Geometry check sheet. Reference: the model listing, model coordinates, mm. A direction names the side the tool comes from. Round coordinates to 2 decimals unless told otherwise and drop trailing zeros. Write each loop counter-clockwise with the first axis right and the second up, starting at its lowest first coordinate (ties: lowest second). Pieces come first, ordered by that corner, then holes. Notation, with made-up numbers: M 34.5,51.5 L 88.5,51.5 A22 ccw 88.5,79.5 Z; hole C -2,2 d4. An arc over 180 degrees is marked long. Use a Markdown table: item, result.
Autodesk Inventor part; units mm, degrees
ref_plane "YZ Plane" through (0, 0, 0) normal (1, 0, 0) x (0, 1, 0)
ref_plane "XZ Plane" through (0, 0, 0) normal (0, 1, 0) x (-1, 0, 0)
ref_plane "XY Plane" through (0, 0, 0) normal (0, 0, 1) x (1, 0, 0)
ref_plane "Arbeitsebene9" through (-58.9003, 150.915, -19.5294) normal (1, 0, 0) x (0, 1, 0.0002861)
ref_plane "Arbeitsebene10" through (-3.3213, 95.2, -15) normal (1, 0, 0) x (0, 1, 0)
sketch "Skizze8" plane through (-3.3213, 95.2, -15) normal (1, 0, 0) x (0, 1, 0)
  line L0 (51.0327, -12.5388) -> (54.3913, -9.7235)
  line L1 (55.2125, -10.1069) -> (55.2018, -30.9624)
  line L2 (54.3802, -31.345) -> (51.0244, -28.5262)
  line L3 (50.2028, -28.9088) -> (50.1999, -34.5321)
  line L4 (50.2154, -4.5321) -> (50.2115, -12.1553)
  line L5 (50.2154, -13.2238) -> (55.2125, -9.0351)
  line L6 (55.2125, -9.0351) -> (55.2125, -32.0442)
  line L7 (55.2125, -32.0442) -> (50.2154, -27.8467)
  line L8 (50.2154, -13.2238) -> (50.2154, -27.8467)
  line L9 (54.9125, -9.678) -> (50.5154, -13.3638)
  line L10 (50.5154, -13.3638) -> (50.5154, -27.7069)
  line L11 (50.5154, -27.7069) -> (54.9125, -31.4004)
  line L12 (54.9125, -31.4004) -> (54.9125, -9.678)
  line L13 (50.5154, -13.3638) -> (46.5154, -13.3638)
  line L14 (50.5154, -13.3638) -> (54.5154, -13.3638) construction
  line L15 (46.5154, -13.3638) -> (46.5154, -27.7069)
  line L16 (46.5154, -27.7069) -> (50.5154, -27.7069)
  line L17 (67.5498, -4.541) -> (50.2154, -4.5321)
  line L18 (61.046, -34.5285) -> (50.2065, -34.5303)
  line L19 (46.5154, -13.3638) -> (49.8154, -13.3638)
  line L20 (49.8154, -13.3638) -> (49.8154, -4.5318)
  line L21 (49.8154, -4.5318) -> (46.5154, -4.5318)
  line L22 (46.5154, -4.5318) -> (46.5154, -13.3638)
  line L23 (46.5154, -27.7069) -> (49.8154, -27.7069)
  line L24 (49.8154, -27.7069) -> (49.8154, -34.5304)
  line L25 (49.8154, -34.5304) -> (46.5154, -34.5304)
  line L26 (46.5154, -34.5304) -> (46.5154, -27.7069)
  point P0 (-95.2, 15)
  point P1 (50.2154, -27.7069)
  point P2 (54.3913, -9.7235)
  point P3 (50.2154, -13.3638)
  dimension "d62" = 0.3
  dimension "d63" = 4
  dimension "d64" = 180
  dimension "d65" = 0.4
extrude "Extrusion5" add sketch "Skizze8" along normal blind 40 contours L13 L10 L16 L8 | L8 L16 L15 L13 | L9 L12 L11 L10 | L13 L22 L21 L20 | L24 L25 L26 L16
sketch "Skizze9" plane through (-3.3213, 150.1125, -5.7071) normal (0, 1, 0) x (1, 0, 0)
  line L0 (10.4, 23.7321) -> (29.6, 23.7321)
  line L1 (29.6, 23.7321) -> (29.6, 35.9321)
  line L2 (29.6, 35.9321) -> (10.4, 35.9321)
  line L3 (10.4, 35.9321) -> (10.4, 23.7321)
  line L4 (10.4, 23.7321) -> (29.6, 35.9321) construction
  line L5 (29.6, 23.7321) -> (10.4, 35.9321) construction
  line L6 (0, 40.6933) -> (0, 18.9709)
  line L7 (0, 18.9709) -> (40, 18.9709)
  line L8 (40, 40.6933) -> (40, 18.9709)
  line L9 (0, 40.6933) -> (40, 40.6933)
  point P0 (3.3213, -5.7071)
  point P1 (20, 29.8321)
  dimension "d52" = 19.2
  dimension "d53" = 12.2
fillet "Rundung3" radius 1 5 edges at (16.6787, 150.1125, -24.678) (16.6787, 150.1125, -46.4004) (16.6787, 145.0154, -42.7069) (16.6787, 145.7154, -28.3638) (16.6787, 145.0154, -28.3638)
hole "Bohrung4" at (7.0787, 150.1125, -29.4392) at (26.2787, 150.1125, -29.4392) at (26.2787, 150.1125, -41.6392) at (7.0787, 150.1125, -41.6392) direction (0, -1, 0) diameter 2.8 end through all counterbore diameter 6 counterbore depth 3.53
ref_plane "Arbeitsebene11" through (-3.3213, 141.7154, -34.5311) normal (0, 0, 1) x (1, 0, 0)
ref_plane "Arbeitsebene12" through (16.6787, 95.2, -15) normal (1, 0, 0) x (0, 0, -1)
properties part number "40_Cube_Z-only_illuminationarm_base-wifiholder_slidermount"
Item 1: Cross-section at C-C, the plane x = 9. Record the cut outline in (y, z), and give its area (3 significant figures).
Outcome:
| item | result |
|---|---|
| outline | M 141.72,-49.53 L 145.02,-49.53 L 145.02,-43.66 A1 cw 145.72,-42.71 L 146.58,-43.44 L 146.58,-39.34 L 150.11,-39.34 L 150.11,-31.74 L 146.58,-31.74 L 146.58,-27.63 A1 cw 145.02,-26.81 L 145.02,-19.53 L 141.72,-19.53 Z; M 147.18,-27.14 L 150.11,-27.14 L 150.11,-26.82 A1 ccw 148.47,-26.05 Z; M 147.19,-43.94 L 148.47,-45.02 A1 ccw 150.11,-44.25 L 150.11,-43.94 Z |
| area | 155 mm2 |
Item 2: Cross-section at B-B, the plane x = 15.5. Record the cut outline in (y, z), and give its area (3 significant figures).
Outcome:
| item | result |
|---|---|
| outline | M 141.72,-49.53 L 145.02,-49.53 L 145.02,-43.66 A1 cw 145.72,-42.71 L 148.47,-45.02 A1 ccw 150.11,-44.25 L 150.11,-26.82 A1 ccw 148.47,-26.05 L 146.66,-27.57 A1 cw 145.02,-26.81 L 145.02,-19.53 L 141.72,-19.53 Z |
| area | 187 mm2 |
Item 3: Material ranges on line 1 along X through (y, z) = (144.25, -41.75); line 2 along Z through (x, y) = (27, 149.5); line 3 along X through (y, z) = (148.25, -31.5), recorded low to high. Write a range as from..to.
Outcome:
| item | result |
|---|---|
| line 1 | x = -3.32..5.68, 8.47..24.88, 27.67..36.68 |
| line 2 | z = -45.18..-44.55, -38.73..-32.35, -26.53..-25.9 |
| line 3 | x = -3.32..4.9, 9.26..24.1, 28.46..36.68 |
Item 4: Go/stop test with flat-tipped pins: pin 1 (2 mm diameter, centred on x = 26.28, z = -29.44, fed in from -Y); pin 2 (1 mm diameter, centred on x = 29, z = -24.5, fed in from +Y); pin 3 (2.5 mm diameter, centred on x = 27, z = -29, fed in from +Y); pin 4 (4.5 mm diameter, centred on x = 14.5, z = -47, fed in from +Y). Record where each tip stops, or that it passes through.
Outcome:
| item | result |
|---|---|
| pin 1 | passes through |
| pin 2 | stops at y = 145.02 |
| pin 3 | stops at y = 146.58 |
| pin 4 | stops at y = 149.98 |
Item 5: Mould release check, pull along Z, two halves, no side actions. Record for faces 1 (the face through (16.399, 147.073, -43.847)), 2 (the face through (6.178, 148.323, -38.778)), 3 (the face through (-3.321, 145, -35)): +Z half, -Z half, draft (parallel to the pull), parting line (faces both ways), or undercut.
Outcome:
| item | result |
|---|---|
| face 1 | -Z half |
| face 2 | undercut |
| face 3 | draft |
Item 6: Access from +Z, -Z, +X, -X, +Y, -Y to the whole of each face (thin tool, end or side, straight path). Record for faces 4 (the face through (26, 146.582, -31)), 5 (the face through (16, 145.015, -47)), 6 (the face through (16, 141.715, -34)), 7 (the face through (16.4, 147.58, -26.8)).
Outcome:
| item | result |
|---|---|
| face 4 | +Y |
| face 5 | -Z, +X, -X |
| face 6 | +Z, -Z, +X, -X, -Y |
| face 7 | +Z, +X, -X |
Item 7: Cross-section at A-A, the plane z = -29.5. Record the cut outline in (x, y), and give its area (3 significant figures).
Outcome:
| item | result |
|---|---|
| outline | M -3.32,141.72 L 5.68,141.72 L 5.68,146.58 L 4.08,146.58 L 4.08,150.11 L -3.32,150.11 Z; M 8.48,141.72 L 24.88,141.72 L 24.88,146.58 L 23.28,146.58 L 23.28,150.11 L 10.08,150.11 L 10.08,146.58 L 8.48,146.58 Z; M 27.68,141.72 L 36.68,141.72 L 36.68,150.11 L 29.28,150.11 L 29.28,146.58 L 27.68,146.58 Z |
| area | 266 mm2 |
Item 8: Cross-section at D-D, the plane y = 143.5. Record the cut outline in (x, z).
Outcome:
| item | result |
|---|---|
| outline | M -3.32,-49.53 L 36.68,-49.53 L 36.68,-19.53 L -3.32,-19.53 Z; hole C 7.08,-41.64 d2.8; hole C 7.08,-29.44 d2.8; hole C 26.28,-41.64 d2.8; hole C 26.28,-29.44 d2.8 |
